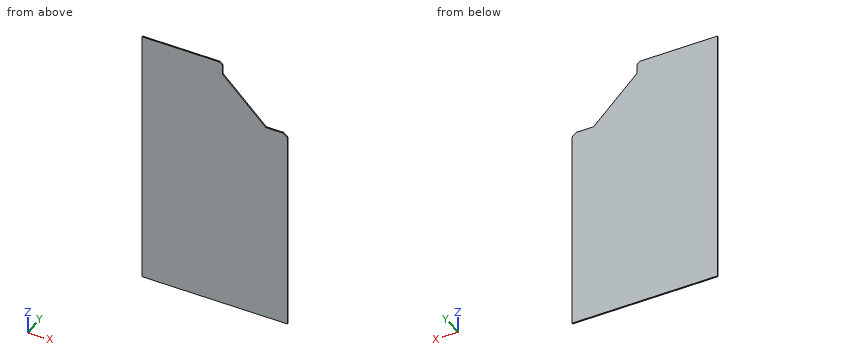
from build123d import *

# Parameters (mm, degrees)
F0_W     = 235
F0_H     = 428
F1_DEPTH = 2
F2_SIZE2 = 96
F2_SIZE  = 110
F4_DEPTH = 25


with BuildPart() as f1:
    # F0 (on Front) → F1 (new body)
    with BuildSketch(Plane.XZ):
        with Locations((-11.5827983245, 118.5401997186)):
            Rectangle(F0_W, F0_H)
    extrude(amount=F1_DEPTH)

    # F2
    f2_edges = [f1.edges().sort_by_distance(p)[0] for p in [
        (105.917202, -1, 332.5402),
    ]]
    f2_side = f1.faces().sort_by_distance((-11.582798, -1, 332.5402))[0]
    chamfer(f2_edges, length=F2_SIZE, length2=F2_SIZE2, reference=f2_side)

    # F3 (on face) → F4 (cut)
    with BuildSketch(Plane.XZ.offset(2)):
        Polygon((99.0422016755, 242.5401997186), (0.9172016755, 328.176563355), (0.9172016755, 312.5401997186), (70.9172016755, 242.5401997186), align=None)
    extrude(amount=-F4_DEPTH, mode=Mode.SUBTRACT)


solid = f1.part
Source: CAD feature listing. Evaluate the final solid. Frame: model axes, mm. Give positions to 0.01 mm unless a question says otherwise; leave off trailing zeros. Order: outer loops, then holes, each group sorted by start corner. A loop starts at its lowest first (then second) coordinate and runs counter-clockwise, first axis right, second up. Notation, with made-up numbers: (-15.75, 84.5) -> (32.25, 84.5) arc R10 cw to (32.25, 103.5) -> close; hole circle Ø5 at (-33, -4). An arc over 180 degrees is marked (long way). Write item = value, one per line.
Q1. Cut plane B-B, the plane x = 90. Output: boundary loops of the cut face in (y, z), and give its area (3 significant figures).
Data:
outline = (-2, -95.46) -> (0, -95.46) -> (0, 242.54) -> (-2, 242.54) -> close
area = 676 mm^2
Q2. Cut plane A-A, the plane y = -0.5. Output: boundary loops of the cut face in (x, z).
Data:
outline = (-129.08, -95.46) -> (105.92, -95.46) -> (105.92, 236.54) -> (99.04, 242.54) -> (70.92, 242.54) -> (0.92, 312.54) -> (0.92, 328.18) -> (-4.08, 332.54) -> (-129.08, 332.54) -> close
Q3. Material intervals for line 1 (Z direction, x = 85, y = -0.2); line 2 (X direction, y = -0.3, z = 261); line 3 (Z direction, x = 42, y = -1.15), sorted ascending. Write a range as from..to.
Data:
line_1 = -95.46..242.54
line_2 = -129.08..52.46
line_3 = -95.46..271.46
Q4. Cut plane C-C, the plane x = 47. Output: boundary loops of the cut face in (y, z), and give its area (3 significant figures).
Data:
outline = (-2, -95.46) -> (0, -95.46) -> (0, 266.46) -> (-2, 266.46) -> close
area = 724 mm^2
Q5. Pin query (flat end, axial travel): pin 1 (0.6 mm diameter, centred on y = -1, z = 317, fed in from +X). Return the tip coordinate at first contact, or that it passes through.
Data:
pin_1 = 0.92
